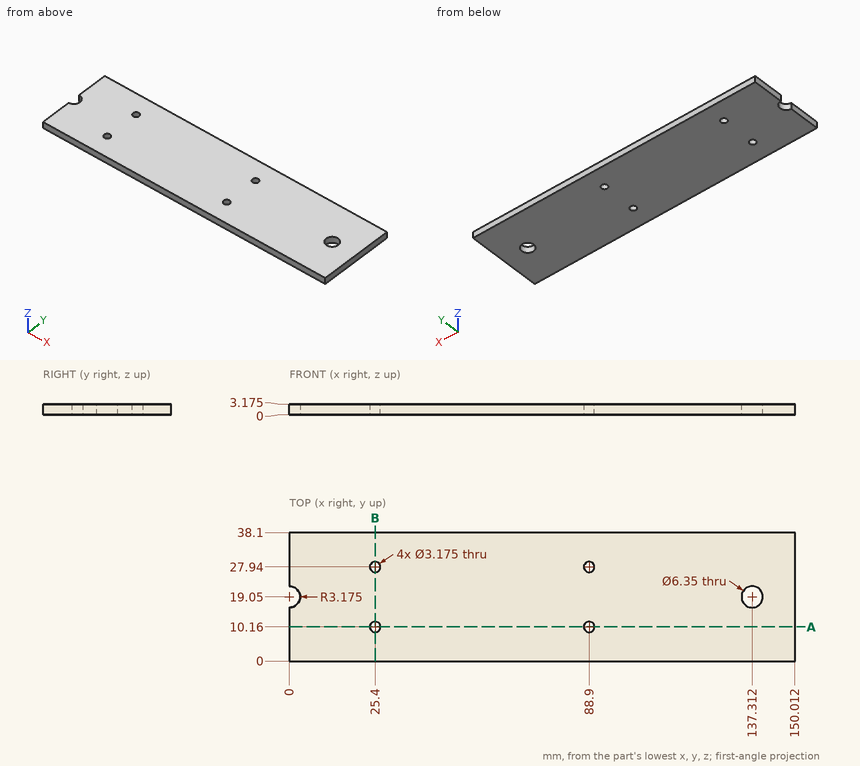
The drawing under review shows one solid part. Ordinate dimensions are in mm from its lowest x, y, z. Coordinates: 2 decimals unless noted, no trailing zeros. Loops run counter-clockwise (first coordinate to the right, second up) from the corner with the lowest first, then second, coordinate; pieces in that order, holes last.
Item 1: Clearance check with a flat-ended pin moving along its axis: pin 1 (6 mm diameter, centred on x = 23, y = 31.5, fed in from -Z). State where the tip first meets the part, or that it passes through.
Completed:
pin 1: stops at z = 0
Item 2: Add section A-A (y = 10.16). Write out the cut boundary in (x, z) (1 decimal), and give its area (3 significant figures).
Completed:
outline: (0, 0) - (23.8, 0) - (23.8, 3.2) - (0, 3.2) - close; (27, 0) - (87.3, 0) - (87.3, 3.2) - (27, 3.2) - close; (90.5, 0) - (150, 0) - (150, 3.2) - (90.5, 3.2) - close
area: 456 mm2
Item 3: Add section B-B (x = 25.4). Write out the cut boundary in (y, z) (1 decimal).
Completed:
outline: (0, 0) - (8.6, 0) - (8.6, 3.2) - (0, 3.2) - close; (11.7, 0) - (26.4, 0) - (26.4, 3.2) - (11.7, 3.2) - close; (29.5, 0) - (38.1, 0) - (38.1, 3.2) - (29.5, 3.2) - close
Item 4: Wall thickness on L1, parallel to Y at x = 25.4, z = 2.2; L2, parallel to X at y = 11, z = 1.65; L3, parallel to Y at x = 26.5, z = 1 (1 decimal): over which ranges is each line inside the solid? List them lowest first.
Completed:
L1: y = 0 to 8.57, 11.75 to 26.35, 29.53 to 38.1
L2: x = 0 to 24.05, 26.75 to 87.55, 90.25 to 150.01
L3: y = 0 to 9, 11.3 to 26.8, 29.1 to 38.1
